Input: part model. Units: mm. Frame: model coordinates. Give positions to 0.01 mm unless a question says otherwise; leave off trailing zeros. Loops run counter-clockwise (first coordinate to the right, second up) from the corner with the lowest first, then second, coordinate; pieces in that order, holes last. Notation, with made-up numbers: M -1,45 L 5,45 A19 cw 5,60 Z; hole C -26,65 d1. An arc over 180 degrees is marked long. One line per item, written item: value. Start each with the question number.
(1) Section D-D on y = -3.75. Output: boundary loops of the cut face in (x, z), plus the area to 3 significant figures.
(2) Ray query, line 1 along X through (y, z) = (-0.5, 0.6); line 2 along Y through (x, z) = (2.5, 3.2). Return the intervals inside material, ascending. Write a range as from..to.
(3) Section A-A on y = 1. Output: boundary loops of the cut face in (x, z).
(4) Pin query (flat end, axial travel): P1, Ø1, axis at y = -1, z = 1, coming from the -X side; P2, Ø0.9, axis at x = -5.5, y = 0, coming from the +Z side. Return the tip coordinate at first contact, or that it passes through.
(5) Pull-direction query (Z, two-part tool) for faces 1 (the flat face through (0, -4, 0)), 2 (the cylindrical face through (-1.164, -4.006, 1.813)), 3 (the flat face through (3, -4, 0.8)), 4 (the flat face through (-0.1, -4.4, 0.6)); classes: released by +Z, released by -Z, zero draft, split by the parting line, or undercut.
(6) Section C-C on z = 0.5. Output: boundary loops of the cut face in (x, y).
(7) Section B-B on x = -3.5. Output: boundary loops of the cut face in (y, z).
```python
from build123d import *

# Parameters (mm, degrees)
F1_DEPTH = 0.8
F3_DEPTH = 0.8


with BuildPart() as f1:
    # F0 (on Top) → F1 (new body)
    with BuildSketch(Plane.XY):
        Polygon((5.75, -4.4), (5.75, 4.4), (4.95, 4.4), (4.95, -3.6), (-4.95, -3.6), (-4.95, 4.4), (-5.75, 4.4), (-5.75, -4.4), align=None)
    extrude(amount=F1_DEPTH)

    # F2 (on face) → F3 (join)
    with BuildSketch(Plane.XZ.offset(4.4)):
        with BuildLine():
            Line((-1.3517540975, 3.4676363777), (-4.4016095807, 3.4676363777))
            ThreePointArc((-4.4016095807, 3.4676363777), (-5.1731426527, 2.2425551298), (-5.2961143665, 0.8))
            Line((-5.2961143665, 0.8), (-4.4836062007, 0.8))
            ThreePointArc((-4.4836062007, 0.8), (-4.4816891927, 1.7839754849), (-4.0488441208, 2.6676363777))
            Line((-4.0488441208, 2.6676363777), (-1.7281457549, 2.6676363777))
            ThreePointArc((-1.7281457549, 2.6676363777), (-1.1580554374, 1.8001751094), (-0.8803113597, 0.8))
            Line((-0.8803113597, 0.8), (0, 0.8))
            ThreePointArc((0, 0.8), (-0.4621715879, 2.2421077724), (-1.3517540975, 3.4676363777))
        make_face()
        with BuildLine():
            ThreePointArc((1.3517540975, 3.4676363777), (0.4621715879, 2.2421077724), (0, 0.8))
            Line((0, 0.8), (0.8803113597, 0.8))
            ThreePointArc((0.8803113597, 0.8), (1.1580554374, 1.8001751094), (1.7281457549, 2.6676363777))
            Line((1.7281457549, 2.6676363777), (4.0488441208, 2.6676363777))
            ThreePointArc((4.0488441208, 2.6676363777), (4.4816891927, 1.7839754849), (4.4836062007, 0.8))
            Line((4.4836062007, 0.8), (5.2961143665, 0.8))
            ThreePointArc((5.2961143665, 0.8), (5.1731426527, 2.2425551298), (4.4016095807, 3.4676363777))
            Line((4.4016095807, 3.4676363777), (1.3517540975, 3.4676363777))
        make_face()
    extrude(amount=-F3_DEPTH)


solid = f1.part
```
Output values:
1. outline: M -5.75,0 L 5.75,0 L 5.75,0.8 L 5.3,0.8 A3.06 ccw 4.4,3.47 L 1.35,3.47 A4.79 ccw 0,0.8 A4.79 ccw -1.35,3.47 L -4.4,3.47 A3.06 ccw -5.3,0.8 L -5.75,0.8 Z; hole M -4.48,0.8 L -0.88,0.8 A3.36 ccw -1.73,2.67 L -4.05,2.67 A2.19 ccw Z; hole M 0.88,0.8 L 4.48,0.8 A2.19 ccw 4.05,2.67 L 1.73,2.67 A3.36 ccw Z
1. area: 21.6 mm²
2. line 1: x = -5.75..-4.95, 4.95..5.75
2. line 2: y = -4.4..-3.6
3. outline: M -5.75,0 L -4.95,0 L -4.95,0.8 L -5.75,0.8 Z; M 4.95,0 L 5.75,0 L 5.75,0.8 L 4.95,0.8 Z
4. P1: stops at x = -5.75
4. P2: stops at z = 0.8
5. face 1: released by -Z
5. face 2: undercut
5. face 3: undercut
5. face 4: zero draft
6. outline: M -5.75,-4.4 L 5.75,-4.4 L 5.75,4.4 L 4.95,4.4 L 4.95,-3.6 L -4.95,-3.6 L -4.95,4.4 L -5.75,4.4 Z
7. outline: M -4.4,0 L -3.6,0 L -3.6,0.8 L -4.4,0.8 Z; M -4.4,2.67 L -3.6,2.67 L -3.6,3.47 L -4.4,3.47 Z
